The figure shows three views and two pictorial views of one solid part (mm, origin at its lowest corner). Answer the questions. Coordinates: 2 decimals unless noted, no trailing zeros. Write each loop counter-clockwise with the first axis right and the second up, starting at its lowest first coordinate (ties: lowest second). Pieces come first, ordered by that corner, then holes.
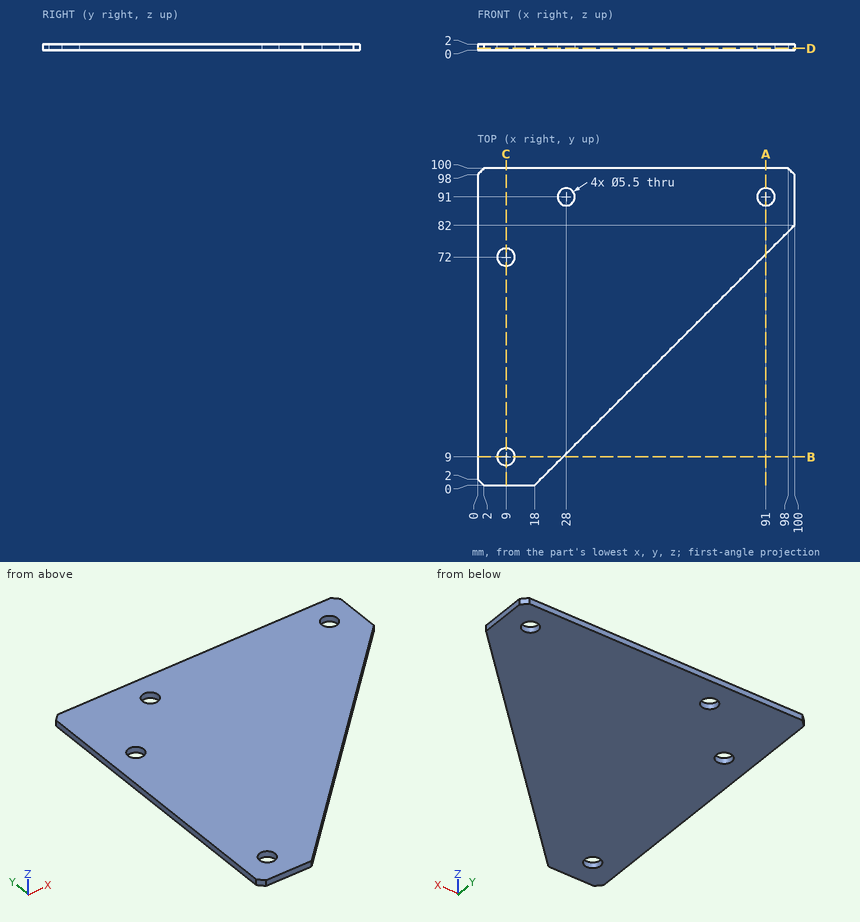
Q1. The part is cut by section C-C, the plane x = 9. Write down the section's boundary in (y, z), then the cut area to 3 significant figures.
Answers below:
outline: (0, 0) - (6.25, 0) - (6.25, 2) - (0, 2) - close; (11.75, 0) - (69.25, 0) - (69.25, 2) - (11.75, 2) - close; (74.75, 0) - (100, 0) - (100, 2) - (74.75, 2) - close
area: 178 mm2
Q2. The part is cut by section D-D, the plane z = 0.6. Write down the section's boundary in (x, y).
Answers below:
outline: (0, 2) - (2, 0) - (18, 0) - (100, 82) - (100, 98) - (98, 100) - (2, 100) - (0, 98) - close; hole circle Ø5.5 at (9, 9); hole circle Ø5.5 at (9, 72); hole circle Ø5.5 at (28, 91); hole circle Ø5.5 at (91, 91)
Q3. Find the intervals of material crossed by probe 1 along X at (y, z) = (90, 0.35); probe 2 along Y at (x, z) = (9, 1.5); probe 3 along Y at (x, z) = (91, 1.5), in increasing order.
Answers below:
probe 1: x = 0 to 25.44, 30.56 to 88.44, 93.56 to 100
probe 2: y = 0 to 6.25, 11.75 to 69.25, 74.75 to 100
probe 3: y = 73 to 88.25, 93.75 to 100
Q4. The part is cut by section B-B, the plane y = 9. Write down the section's boundary in (x, z), then the cut area to 3 significant figures.
Answers below:
outline: (0, 0) - (6.25, 0) - (6.25, 2) - (0, 2) - close; (11.75, 0) - (27, 0) - (27, 2) - (11.75, 2) - close
area: 43.0 mm2
Q5. Given pin 1 (4.5 mm diameter, centred on x = 9, y = 72, fed in from +Z); pin 2 (4 mm diameter, centred on x = 75, y = 60, fed in from -Z), each flat-ended and moving along its own axis, determine where each tip first touches the part or whether it passes through.
Answers below:
pin 1: passes through
pin 2: stops at z = 0
Q6. The part is cut by section A-A, the plane x = 91. Write down the section's boundary in (y, z).
Answers below:
outline: (73, 0) - (88.25, 0) - (88.25, 2) - (73, 2) - close; (93.75, 0) - (100, 0) - (100, 2) - (93.75, 2) - close
